Here's how the part is built. I have some questions about the finished solid (model axes, mm). A direction names the side the tool comes from. Give positions to 0.01 mm unless a question says otherwise; leave off trailing zeros. Loops run counter-clockwise (first coordinate to the right, second up) from the corner with the lowest first, then second, coordinate; pieces in that order, holes last. Notation, with made-up numbers: (-1.75, 89) - (46.25, 89) arc R28 cw to (46.25, 115) - close; hole circle Ø8 at (69, -40). An arc over 180 degrees is marked (long way). Put each result on its own line as item: value. Start each with the question number.
Autodesk Inventor part; units mm, degrees
ref_plane "YZ Plane" through (0, 0, 0) normal (1, 0, 0) x (0, 1, 0)
ref_plane "XZ Plane" through (0, 0, 0) normal (0, 1, 0) x (-1, 0, 0)
ref_plane "XY Plane" through (0, 0, 0) normal (0, 0, 1) x (1, 0, 0)
sketch "Sketch1" plane through (0, 0, 0) normal (0, 0, 1) x (1, 0, 0)
  circle A0 centre (0, 0) radius 30.5
  circle A1 centre (141.8, 0) radius 60.5
  line L0 (129.0003, 59.1305) -> (-6.4528, 29.8096)
  line L1 (-6.4528, -29.8096) -> (129.0003, -59.1305)
  line L2 (60, 44.1943) -> (60, -44.1943)
  dimension "d0" = 61
  dimension "d1" = 121
  dimension "d2" = 141.8
  dimension "d3" = 60
extrude "Extrusion1" add sketch "Sketch1" against normal blind 8.25 contours A0 | A0 L0 L2 L1
shell "Shell1" thickness 4 removed faces 1 at (37.8491, -9.9365, -8.25)
sketch "Sketch6" plane through (0, 0, 0) normal (0, 0, 1) x (1, 0, 0)
  point P0 (0, 0)
  point P1 (0, 0)
hole "Hole3" at (0, 0, 0) direction (0, 0, -1) diameter 30 end through all
sketch "Sketch12" plane through (0, 0, 0) normal (0, 0, 1) x (1, 0, 0)
  circle A0 centre (0, 0) radius 45
  circle A1 centre (0, 0) radius 15
  circle A2 centre (0, 0) radius 15
  dimension "d55" = 90
extrude "Extrusion5" add sketch "Sketch12" against normal blind 4
sketch "Sketch7" plane through (56, -39.2358, -4) normal (0, 0, -1) x (-1, 0, 0)
  line L0 (26.9325, 5.83) -> (-25.6804, -5.5589)
  line L1 (-25.6804, -5.5589) -> (-25.6804, 84.0306)
  line L2 (-25.6804, 84.0306) -> (28.864, 72.2236)
  line L3 (28.864, 72.2236) -> (24.7276, 5.3527)
  line L4 (61.6065, 13.3357) -> (0, 0)
  line L5 (0, 78.4716) -> (61.6065, 65.136)
  point P0 (56, 39.2358)
extrude "Extrusion2" cut sketch "Sketch7" along normal through all
sketch "Sketch8" plane through (-5.6065, 25.9001, -8.25) normal (0.2115656, -0.9773638, 0) x (0.9773638, 0.2115656, 0)
  line L0 (0, 4.25) -> (0, 0)
  line L1 (67.126, 0) -> (0, 0)
  line L2 (0, 4.25) -> (8, 4.25)
  line L3 (8, 4.25) -> (8, 0)
  line L4 (8, 0) -> (0, 0)
  line L5 (0, 0) -> (0, 4.25)
  line L6 (53, 4.25) -> (61, 4.25)
  line L7 (61, 4.25) -> (61, 0)
  line L8 (61, 0) -> (53, 0)
  line L9 (53, 0) -> (53, 4.25)
  point P0 (0, 8.25)
  dimension "d33" = 8
  dimension "d34" = 8
  dimension "d35" = 45
extrude "Extrusion3" add sketch "Sketch8" along normal blind 4
sketch "Sketch9" plane through (0, 0, -8.25) normal (0, 0, -1) x (-1, 0, 0)
  line L0 (4.7602, 21.9907) -> (-3.0587, 23.6832)
  line L1 (-60, 44.1943) -> (-25.8853, 36.8097)
  line L2 (-46.1938, 37.1131) -> (-47.0401, 33.2037)
  line L3 (-47.0401, 33.2037) -> (-53.1727, 42.6863)
  line L4 (-1.3662, 31.5021) -> (4.7602, 21.9907)
  line L5 (-3.0587, 23.6832) -> (6.4528, 29.8096)
  line L6 (-47.0401, 33.2037) -> (-54.859, 34.8962)
  line L7 (-54.859, 34.8962) -> (-45.3475, 41.0226)
  point P0 (0, 0)
  point P1 (-50.1032, 37.9594)
  point P2 (1.697, 26.7464)
hole "Hole4" at (50.1032, 37.9594, -8.25) at (-1.697, 26.7464, -8.25) direction (0, 0, 1) diameter 3.4 end through all
sketch "Sketch10" plane through (0, 0, 0) normal (0, 0, 1) x (1, 0, 0)
  circle A0 centre (50.1032, 37.9594) radius 1.7
  circle A1 centre (-1.697, 26.7464) radius 1.7
  point P0 (0, 0)
hole "Hole5" at (50.1032, 37.9594, 0) at (-1.697, 26.7464, 0) direction (0, 0, -1) diameter 6 depth 4
mirror "Mirror1" about plane through (0, 0, 0) normal (0, 1, 0) of "Extrusion3", "Hole4", "Hole5"
sketch "Sketch13" plane through (0, 0, -4) normal (0, 0, -1) x (-1, 0, 0)
  line L0 (0, -40) -> (-34.641, -20)
  line L1 (-34.641, -20) -> (-34.641, 20)
  line L2 (-34.641, 20) -> (0, 40)
  line L3 (0, 40) -> (34.641, 20)
  line L4 (34.641, 20) -> (34.641, -20)
  line L5 (34.641, -20) -> (0, -40)
  point P0 (0, 0)
  point P1 (0, 0)
  dimension "d59" = 80
hole "Hole6" at (34.641, -20, -4) at (0, -40, -4) at (-34.641, -20, -4) at (-34.641, 20, -4) at (0, 40, -4) at (34.641, 20, -4) direction (0, 0, 1) diameter 3.4 end through all
equation "\"d34\" = d33"
properties part number "J1-sketch"
1) Suppose I cut it at A-A on y = 0. Please give me the cut outline in (x, z), plus the area to 3 significant figures.
2) Thinking about a two-plate mould opening in X: for faces 1 (the flat face through (-31, -3, -4)), 2 (the flat face through (54.43, -36.88, -6.15)), 3 (the flat face through (46.61, -35.19, -6.1)), which applies, pulls with the +X half, pulls with the -X half, needs draft (parallel to the pull), parting line crosses it, or undercut?
3) Suppose I cut it at D-D on y = -20. Please give me the cut outline in (x, z).
4) I'm going to push flat-ended pins straight in: P1, Ø3, axis at x = 45.5, z = -1, coming from the +Y side; P2, Ø1.5, axis at x = 30.5, z = -6.5, coming from the +Y side; P3, Ø3, axis at x = -0.5, y = -27, coming from the +Z side. Where does each tip first touch, or does it pass through?
5) Which directions (+Z, -Z, +X, -X, +Y, -Y) give clear straight access to the entire face, cutting with the end or side of a thin tool? Please do faces 4 (the flat face through (51.4, -39.3, -4)), 5 (the cylindrical face through (-26.495, 0.504, -6.095)), 6 (the flat face through (-0.906, 22.825, -6.095)).
6) Suppose I cut it at B-B on z = -2.25. Give the number of separate pieces and of enclosed holes in the cut face, plus the area to 3 significant figures.
7) I need wall thicknesses on line 1 (X direction, y = 20, z = -3.1); line 2 (X direction, y = -21.5, z = -3.25); line 3 (Z direction, x = -32.5, y = -19). Which ranges of each line are inside material? Lowest first, please.
8) Suppose I cut it at C-C on x = -19. Please give me the cut outline in (y, z).
Ans:
1. outline: (-45, -4) - (-30.5, -4) - (-30.5, -8.25) - (-26.5, -8.25) - (-26.5, -4) - (-15, -4) - (-15, 0) - (-45, 0) - close; (15, -4) - (60, -4) - (60, 0) - (15, 0) - close
1. area: 317 mm²
2. face 1: needs draft
2. face 2: pulls with the +X half
2. face 3: undercut
3. outline: (-40.31, -4) - (-36.34, -4) - (-36.34, 0) - (-40.31, 0) - close; (-32.94, -4) - (-23.03, -4) - (-23.03, -8.25) - (-17.39, -8.25) - (-17.39, -4) - (32.94, -4) - (32.94, 0) - (-32.94, 0) - close; (36.34, -4) - (60, -4) - (60, 0) - (36.34, 0) - close
4. P1: stops at y = 41.38
4. P2: stops at y = 37.97
4. P3: stops at z = -4
5. face 4: +Z
5. face 5: -Z
5. face 6: -Z, +X
6. separate pieces: 1
6. enclosed holes: 11
6. area: 7,260 mm²
7. line 1: x = -40.31 to -36.34, -32.94 to 32.94, 36.34 to 60
7. line 2: x = -39.53 to -35.44, -33.84 to 33.84, 35.44 to 60
7. line 3: z = -4 to 0
8. outline: (-40.79, -4) - (-23.86, -4) - (-23.86, -8.25) - (-18.47, -8.25) - (-18.47, -4) - (18.47, -4) - (18.47, -8.25) - (23.86, -8.25) - (23.86, -4) - (40.79, -4) - (40.79, 0) - (-40.79, 0) - close
